Model file for the job. Use its own axes, mm. Round coordinates to 2 decimals unless told otherwise and drop trailing zeros. Write each loop counter-clockwise with the first axis right and the second up, starting at its lowest first coordinate (ties: lowest second). Pieces come first, ordered by that corner, then holes.
```python
from build123d import *

# Parameters (mm, degrees)
SKETCH_1_R               = 3
EXTRUDE_1_DEPTH          = 4
SKETCH_2_R               = 1.5
CUT_EXTRUDE_1_DEPTH      = 4
PATTERN_CIRCULAR_1_COUNT = 4


with BuildPart() as part:
    # 草图1 → 凸台-拉伸1 (new body)
    with BuildSketch(Plane(origin=(0, 0, 0), x_dir=(1, 0, 0), z_dir=(0, 1, 0))):
        with BuildLine():
            Line((-111.375, 10), (111.375, 10))
            ThreePointArc((111.375, 10), (121.375, 0), (111.375, -10))
            Line((111.375, -10), (-111.375, -10))
            ThreePointArc((-111.375, -10), (-121.375, 0), (-111.375, 10))
        make_face()
        with Locations(Location((-111.375, 0, 0), (0, 0, 270))):
            Circle(SKETCH_1_R, mode=Mode.SUBTRACT)
        with Locations(Location((111.375, 0, 0), (0, 0, 270))):
            Circle(SKETCH_1_R, mode=Mode.SUBTRACT)
    extrude(amount=EXTRUDE_1_DEPTH)

    # 草图2 → 切除-拉伸1 (cut)
    with BuildSketch(Plane(origin=(0, 4, 0), x_dir=(1, 0, 0), z_dir=(0, 1, 0))):
        with Locations(Location((-111.375, 6.5, 0), (0, 0, 270))):
            Circle(SKETCH_2_R)
    cut_extrude_1 = extrude(amount=-CUT_EXTRUDE_1_DEPTH, mode=Mode.SUBTRACT)

    # 阵列(圆周)1: 切除-拉伸1 ×4 about axis
    pattern_circular_1_axis = Axis((-111.375, 0, 0), (0, 1, 0))
    for i in range(1, PATTERN_CIRCULAR_1_COUNT):
        add(cut_extrude_1.rotate(pattern_circular_1_axis, i * 360 / PATTERN_CIRCULAR_1_COUNT), mode=Mode.SUBTRACT)


solid = part.part
```
1) Wall check: probe 1 along X at (y, z) = (1.05, 0) (3 decimals); probe 2 along X at (y, z) = (2.5, 2.75); probe 3 along X at (y, z) = (3.6, -2.25). Give the ranges that are in metal, low to high.
2) Pull direction X, two halves, no side cores. Call faces 1 (the face through (2, 4, 0)), 2 (the face through (121.373, 1.972, -0.22)), 3 (the face through (-121.373, 1.972, 0.22)), 4 (the face through (113.403, 1.972, -2.211)): released by +X, released by -X, zero draft, split by the parting line, or undercut.
3) Cut at A-A on y = 0.7. List the corners of the cut face in (x, z) (3 decimals).
4) Flat gauge pin, fed straight in: pin 1 Ø2.5 at (x, z) = (-104.875, 0) entering from -Y. Where does the tip first touch, or does it go through?
Result sheet:
1. probe 1: x = -121.375 to -119.375, -116.375 to -114.375, -108.375 to -106.375, -103.375 to 108.375, 114.375 to 121.375
1. probe 2: x = -120.99 to -112.57, -110.18 to 110.18, 112.57 to 120.99
1. probe 3: x = -121.12 to -113.36, -109.39 to 109.39, 113.36 to 121.12
2. face 1: zero draft
2. face 2: released by +X
2. face 3: released by -X
2. face 4: undercut
3. outline: (-111.375, -10) - (111.375, -10) arc R10 ccw to (111.375, 10) - (-111.375, 10) arc R10 ccw to start; hole circle Ø3 at (-117.875, 0); hole circle Ø6 at (-111.375, 0); hole circle Ø3 at (-111.375, -6.5); hole circle Ø3 at (-111.375, 6.5); hole circle Ø3 at (-104.875, 0); hole circle Ø6 at (111.375, 0)
4. pin 1: passes through
